Design review of the part built by this model. Coordinates are the model's own, in mm. Face numbers are marked on the shaded views. A direction names the side the tool comes from. Give positions to 0.01 mm unless a question says otherwise; leave off trailing zeros. Loops run counter-clockwise (first coordinate to the right, second up) from the corner with the lowest first, then second, coordinate; pieces in that order, holes last. Notation, with made-up numbers: M 67.25,19 L 95.25,19 A16 cw 95.25,32 Z; hole C 75,33.5 d2. An arc over 180 degrees is marked long. Answer as CSV lines item,"result".
```python
from build123d import *
from build123d.topology import SkipClean

# Parameters (mm, degrees)
SKETCH1_R               = 17.5
BOSS_EXTRUDE1_DEPTH     = 5
SKETCH3_R               = 20.5
SKETCH3_R_2             = 17.5
BOSS_EXTRUDE3_DEPTH     = 1
BOSS_EXTRUDE2_OUTLINE_R = 7.5
BOSS_EXTRUDE2_DEPTH     = 0.5
SKETCH4_R               = 8
BOSS_EXTRUDE5_DEPTH     = 2
BOSS_EXTRUDE6_START     = 7
SKETCH5_R               = 4
BOSS_EXTRUDE6_DEPTH     = 7
CHAMFER1_SIZE           = 1


# Read off the part's stored shape, not the designer's step: Boss-Extrude2
with BuildPart() as part:
    # Sketch1 → Boss-Extrude1 (new, symmetric)
    with BuildSketch(Plane.XY):
        with Locations((-4, 0)):
            Circle(SKETCH1_R)
        with BuildLine():
            Line((1.5, 3.708099244), (1.5, -3.708099244))
            ThreePointArc((1.5, -3.708099244), (-4, 0), (1.5, 3.708099244))
        make_face(mode=Mode.SUBTRACT)
    extrude(amount=BOSS_EXTRUDE1_DEPTH, both=True)

    # Sketch3 → Boss-Extrude3 (add)
    # profile 1 of 2: a face of its own
    with SkipClean():  # the faces are left unmerged after this step: merging them gives an invalid solid
        with BuildSketch(Plane(origin=(0, 0, -5), x_dir=(-1, 0, 0), z_dir=(0, 0, -1))):
            with Locations((4, 0)):
                Circle(SKETCH3_R)
            with Locations(Location((4, 0, 0), (0, 0, 180))):
                Circle(SKETCH3_R_2, mode=Mode.SUBTRACT)
        # profile 2 of 2: a face of its own
        with BuildSketch(Plane(origin=(0, 0, -5), x_dir=(-1, 0, 0), z_dir=(0, 0, -1))):
            with Locations(Location((4, 0, 0), (0, 0, 180))):
                Circle(SKETCH3_R_2)
            with BuildLine():
                Line((-1.5, -3.708099244), (-1.5, 3.708099244))
                ThreePointArc((-1.5, 3.708099244), (4, 0), (-1.5, -3.708099244))
            make_face(mode=Mode.SUBTRACT)
        extrude(amount=BOSS_EXTRUDE3_DEPTH)

    # Boss-Extrude2 outline → Boss-Extrude2 (add)
    with SkipClean():  # the faces are left unmerged after this step: merging them gives an invalid solid
        with BuildSketch(Plane(origin=(0, 0, -6), x_dir=(-1, 0, 0), z_dir=(0, 0, -1))):
            Circle(BOSS_EXTRUDE2_OUTLINE_R)
            with BuildLine():
                ThreePointArc((-1.5, 3.708099244), (4, 0), (-1.5, -3.708099244))
                Line((-1.5, -3.708099244), (-1.5, 3.708099244))
            make_face(mode=Mode.SUBTRACT)
        extrude(amount=BOSS_EXTRUDE2_DEPTH)

    # Sketch4 → Boss-Extrude5 (add)
    with SkipClean():  # the faces are left unmerged after this step: merging them gives an invalid solid
        with BuildSketch(Plane.XY.offset(5)):
            Circle(SKETCH4_R)
        extrude(amount=BOSS_EXTRUDE5_DEPTH)

    # Sketch5 → Boss-Extrude6 (add)
    with SkipClean():  # the faces are left unmerged after this step: merging them gives an invalid solid
        with BuildSketch(Plane.XY.offset(7).offset(BOSS_EXTRUDE6_START)):
            Circle(SKETCH5_R)
        extrude(amount=-BOSS_EXTRUDE6_DEPTH)

    # Chamfer1
    chamfer1_edges = [part.edges().sort_by_distance(p)[0] for p in [
        (-8, 0, 7),
    ]]
    chamfer(chamfer1_edges, length=CHAMFER1_SIZE)


solid = part.part
```
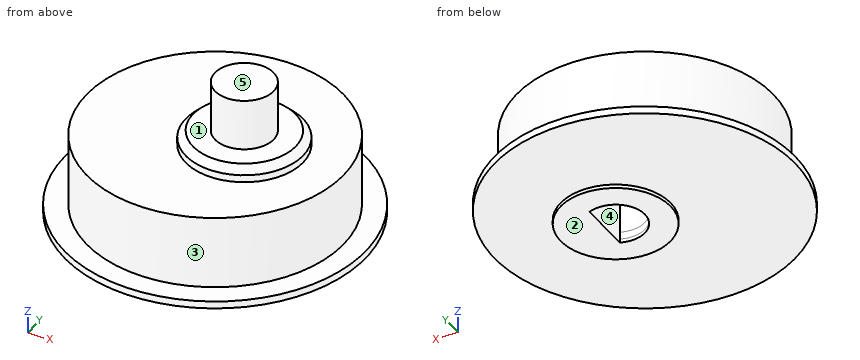
1. We need section D-D, the plane z = 11.5. Write out the cut boundary in (x, y).
Answer block:
outline,"C 0,0 d8"
2. We need section A-A, the plane y = 0. Write out the cut boundary in (x, z), plus the area to 3 significant figures.
Answer block:
outline,"M -24.5,-6 L -7.5,-6 L -7.5,-6.5 L -4,-6.5 L -4,5 L 1.5,5 L 1.5,-6.5 L 7.5,-6.5 L 7.5,-6 L 16.5,-6 L 16.5,-5 L 13.5,-5 L 13.5,5 L 8,5 L 8,6 L 7,7 L 4,7 L 4,14 L -4,14 L -4,7 L -7,7 L -8,6 L -8,5 L -21.5,5 L -21.5,-5 L -24.5,-5 Z"
area,"422 mm²"
3. We need section C-C, the plane z = 2. Write out the cut boundary in (x, y).
Answer block:
outline,"C -4,0 d35; hole M 1.5,-3.71 L 1.5,3.71 A4 ccw long Z"
4. To check wall thickness, follow L1, parallel to Z at x = 1.5, y = 8; L2, parallel to Y at x = 0, z = -5.3; L3, parallel to Z at x = 3.5, y = -2. State the ranges of each line that lie inside material, in increasing order. Write a range as [from, to].
Answer block:
L1,"[-6, 5]"
L2,"[-20.11, -4], [4, 20.11]"
L3,"[-6.5, 7]"
5. For the marked faces 1 and 2, list the 3-axis set-ups (+Z, -Z, +X, -X, +Y, -Y) from which the entire face can be reached by the end or side of a thin tool; tool diameter is ignored.
Answer block:
face 1,"+Z"
face 2,"-Z, +X, -X, +Y, -Y"
6. For P1, Ø5, axis at x = -13, z = 3, coming from the -Y side; P2, Ø3, axis at x = -1.5, y = -1.5, coming from the -Z side; P3, Ø1, axis at x = -18.5, y = -4, coming from the -Z side, all flat-tipped, find the tip position at first contact; note any pin that passes through.
Answer block:
P1,"y = -16.25"
P2,"z = 5"
P3,"z = -6"
7. The part is to be moulded in two halves that separate along X. For the marked faces 3, 4 and 5, say which applies: pulls with the +X half, pulls with the -X half, needs draft (parallel to the pull), parting line crosses it, or undercut.
Answer block:
face 3,"parting line crosses it"
face 4,"undercut"
face 5,"needs draft"
8. We need section B-B, the plane x = 0. Write out the cut boundary in (y, z), plus the area to 3 significant figures.
Answer block:
outline,"M -20.11,-6 L -7.5,-6 L -7.5,-6.5 L -4,-6.5 L -4,5 L 4,5 L 4,-6.5 L 7.5,-6.5 L 7.5,-6 L 20.11,-6 L 20.11,-5 L 17.04,-5 L 17.04,5 L 8,5 L 8,6 L 7,7 L 4,7 L 4,14 L -4,14 L -4,7 L -7,7 L -8,6 L -8,5 L -17.04,5 L -17.04,-5 L -20.11,-5 Z"
area,"383 mm²"
